For this review, take the finished solid that the model builds, in its own axes (mm). Face numbers are marked on the shaded views. Round coordinates to 2 decimals unless told otherwise and drop trailing zeros. Loops run counter-clockwise (first coordinate to the right, second up) from the corner with the lowest first, then second, coordinate; pieces in that order, holes last.
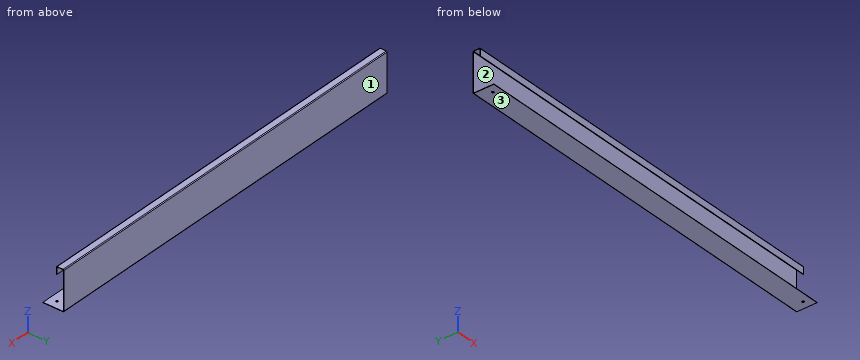
```python
from build123d import *

# Parameters (mm, degrees)
BASE_FLANGE1_DEPTH = 1063
SKETCH2_R          = 3
CUT_EXTRUDE1_DEPTH = 10


# Sheet-metal steps are written as plain solids
with BuildPart() as part:
    # Sketch1 → Base-Flange1 (new body)
    with BuildSketch(Plane(origin=(0, 0, 0), x_dir=(0, 0, -1), z_dir=(1, 0, 0))):
        with BuildLine():
            Line((104, -27.232585832), (104, 26.767414168))
            ThreePointArc((104, 26.767414168), (103.707106781, 27.474520949), (103, 27.767414168))
            Line((103, 27.767414168), (1, 27.767414168))
            ThreePointArc((1, 27.767414168), (0.292893219, 27.474520949), (0, 26.767414168))
            Line((0, 26.767414168), (0, 10.767414168))
            ThreePointArc((0, 10.767414168), (0.292893219, 10.060307386), (1, 9.767414168))
            Line((1, 9.767414168), (19, 9.767414168))
            Line((19, 9.767414168), (19, 8.767414168))
            Line((19, 8.767414168), (1, 8.767414168))
            ThreePointArc((1, 8.767414168), (-0.414213562, 9.353200605), (-1, 10.767414168))
            Line((-1, 10.767414168), (-1, 26.767414168))
            ThreePointArc((-1, 26.767414168), (-0.414213562, 28.18162773), (1, 28.767414168))
            Line((1, 28.767414168), (103, 28.767414168))
            ThreePointArc((103, 28.767414168), (104.414213562, 28.18162773), (105, 26.767414168))
            Line((105, 26.767414168), (105, -27.232585832))
            Line((105, -27.232585832), (104, -27.232585832))
        make_face()
    extrude(amount=BASE_FLANGE1_DEPTH)

    # Sketch2 → Cut-Extrude1 (cut)
    with BuildSketch(Plane.XY.offset(-104)):
        with Locations((21.5, -7.232585832)):
            Circle(SKETCH2_R)
        with Locations((1041.5, -7.232585832)):
            Circle(SKETCH2_R)
    extrude(amount=-CUT_EXTRUDE1_DEPTH, mode=Mode.SUBTRACT)


solid = part.part
```
(1) Insertion check: pin 1 Ø12 at (x, y) = (893.5, -6) entering from +Z; pin 2 Ø6 at (x, z) = (784, -39) entering from -Y; pin 3 Ø14.5 at (x, z) = (555, -8.5) entering from -Y. Each pin has a flat end and moves straight along its axis. Give the tip position at first contact, or say it passes through.
(2) The part is to be moulded in two halves that separate along Z. For the marked faces 1, 2 and 3, say which applies: pulls with the +Z half, pulls with the -Z half, needs draft (parallel to the pull), parting line crosses it, or undercut.
(3) Add section A-A (x = 849). Give the boundary of the cut face in (y, z).
(4) Add section B-B (z = -44.5). Give the boundary of the cut face in (x, y).
(5) For L1, parallel to Z at x = 674, y = 16; L2, parallel to Y at x = 21.5, z = -104.6; L3, parallel to Z at x = 652, y = 5, list the stretches that pass through material, from the lowest coordinate up.
Outcome:
1. pin 1: stops at z = -104
1. pin 2: stops at y = 27.77
1. pin 3: stops at y = 8.77
2. face 1: needs draft
2. face 2: undercut
2. face 3: pulls with the -Z half
3. outline: (-27.23, -105) - (26.77, -105) arc R2 ccw to (28.77, -103) - (28.77, -1) arc R2 ccw to (26.77, 1) - (10.77, 1) arc R2 ccw to (8.77, -1) - (8.77, -19) - (9.77, -19) - (9.77, -1) arc R1 cw to (10.77, 0) - (26.77, 0) arc R1 cw to (27.77, -1) - (27.77, -103) arc R1 cw to (26.77, -104) - (-27.23, -104) - close
4. outline: (0, 27.77) - (1063, 27.77) - (1063, 28.77) - (0, 28.77) - close
5. L1: z = -105 to -104, 0 to 1
5. L2: y = -27.23 to -10.23, -4.23 to 27.97
5. L3: z = -105 to -104
